from build123d import *

# Parameters (mm, degrees)
BOSS_EXTRUDE1_DEPTH = 12
BOSS_EXTRUDE2_DEPTH = 3
FILLET1_R           = 1
SKETCH3_R           = 1.75
CUT_EXTRUDE2_DEPTH  = 3


with BuildPart() as part:
    # Sketch1 → Boss-Extrude1 (new body)
    with BuildSketch(Plane.XY):
        Polygon((-30.5, 3), (-18.5, 3), (-18.5, 15), (18.5, 15), (18.5, 3), (30.5, 3), (30.5, 0), (15.5, 0), (15.5, 12), (-15.5, 12), (-15.5, 0), (-30.5, 0), align=None)
    extrude(amount=-BOSS_EXTRUDE1_DEPTH)

    # Sketch2 → Boss-Extrude2 (add)
    with BuildSketch(Plane.XY):
        Polygon((-18.5, 15), (-10.5, 15), (-10.5, 0), (-30.5, 0), (-30.5, 3), (-18.5, 3), align=None)
        Polygon((30.5, 0), (10.5, 0), (10.5, 15), (18.5, 15), (18.5, 3), (30.5, 3), align=None)
    extrude(amount=BOSS_EXTRUDE2_DEPTH)

    # Fillet1
    fillet1_edges = [part.edges().sort_by_distance(p)[0] for p in [
        (-15.5, 6, -12),
        (-30.5, 3, -4.5),
        (-18.5, 3, -4.5),
        (-18.5, 15, -4.5),
        (15.5, 6, -12),
        (18.5, 15, -4.5),
        (18.5, 3, -4.5),
        (30.5, 3, -4.5),
        (30.5, 1.5, -12),
        (24.5, 3, -12),
        (18.5, 9, -12),
        (-10.5, 15, 1.5),
        (-18.5, 9, 3),
        (-24.5, 3, 3),
        (-30.5, 1.5, 3),
        (-10.5, 7.5, 3),
        (-14.5, 15, 3),
        (0, 15, -12),
        (-18.5, 9, -12),
        (-24.5, 3, -12),
        (-30.5, 1.5, -12),
        (0, 15, 0),
        (10.5, 15, 1.5),
        (30.5, 1.5, 3),
        (24.5, 3, 3),
        (18.5, 9, 3),
        (14.5, 15, 3),
        (10.5, 7.5, 3),
    ]]
    fillet(fillet1_edges, radius=FILLET1_R)

    # Sketch3 → Cut-Extrude2 (cut)
    with BuildSketch(Plane(origin=(0, 3, 0), x_dir=(1, 0, 0), z_dir=(0, 1, 0))):
        with Locations((-24.5, 4.5)):
            Circle(SKETCH3_R)
        with Locations((24.5, 4.5)):
            Circle(SKETCH3_R)
    extrude(amount=-CUT_EXTRUDE2_DEPTH, mode=Mode.SUBTRACT)


solid = part.part
Design review of the part built by this model. Coordinates are the model's own, in mm. A direction names the side the tool comes from. Coordinates: 2 decimals unless noted, no trailing zeros. Order: outer loops, then holes, each group sorted by start corner. A loop starts at its lowest first (then second) coordinate and runs counter-clockwise, first axis right, second up.
Item 1: Take a section at D-D, the plane z = -7. Write out the cut boundary in (x, y), then the cut area to 3 significant figures.
Item 2: For faces 1 (the cylindrical face through (-10.801, 14.715, 0.854)), 2 (the cylindrical face through (15.785, 6.084, -11.699)), 3 (the cylindrical face through (18.215, 8.93, 2.699)), 4 (the flat face through (23, 3, -3)), list the 3-axis set-ups (+Z, -Z, +X, -X, +Y, -Y) from which the entire face can be reached by the end or side of a thin tool; tool diameter is ignored.
Item 3: For pin 1 Ø1 at (x, y) = (-1, 12.5) entering from +Z; pin 2 Ø4 at (y, z) = (8, -5) entering from +X; pin 3 Ø5 at (y, z) = (8, 1.5) entering from -X; pin 4 Ø3 at (x, z) = (24.5, -4.5) entering from +Y, all flat-tipped, find the tip position at first contact; note any pin that passes through.
Item 4: Take a section at C-C, the plane x = 24.5. Write out the cut boundary in (y, z).
Item 5: Take a section at A-A, the plane z = -4.5. Write out the cut boundary in (x, y), then the cut area to 3 significant figures.
Item 6: Take a section at B-B, the plane y = 5.75. Write out the cut boundary in (x, z), then the cut area to 3 significant figures.
Item 7: The part is to be moulded in two halves that separate along X. For faces 5 (the cylindrical face through (24.57, 2.715, -11.699)), 6 (the cylindrical face through (-18.215, 9.07, 2.699)), 7 (the flat face through (0, 12, -6)), say which applies: pulls with the +X half, pulls with the -X half, needs draft (parallel to the pull), parting line crosses it, or undercut.
Item 8: For line 1 (X direction, y = 0.8, z = -4.5); line 2 (Z direction, x = 24.5, y = 0.9); line 3 (X direction, y = 9.5, z = 1.5), list the stretches that pass through material, from the lowest coordinate up.
The answers:
1. outline: (-30.5, 0) - (-15.5, 0) - (-15.5, 12) - (15.5, 12) - (15.5, 0) - (30.5, 0) - (30.5, 2) arc R1 ccw to (29.5, 3) - (19.5, 3) arc R1 cw to (18.5, 4) - (18.5, 14) arc R1 ccw to (17.5, 15) - (-17.5, 15) arc R1 ccw to (-18.5, 14) - (-18.5, 4) arc R1 cw to (-19.5, 3) - (-29.5, 3) arc R1 ccw to (-30.5, 2) - close
1. area: 255 mm2
2. face 1: +Z, +Y
2. face 2: -Z, -Y
2. face 3: +Z, +X, +Y
2. face 4: +Z, -Z, +X, +Y
3. pin 1: stops at z = 0
3. pin 2: stops at x = 18.5
3. pin 3: stops at x = -18.5
3. pin 4: passes through
4. outline: (0, -12) - (2, -12) arc R1 ccw to (3, -11) - (3, -6.25) - (0, -6.25) - close; (0, -2.75) - (3, -2.75) - (3, 2) arc R1 ccw to (2, 3) - (0, 3) - close
5. outline: (-30.5, 0) - (-26.25, 0) - (-26.25, 3) - (-29.5, 3) arc R1 ccw to (-30.5, 2) - close; (-22.75, 0) - (-15.5, 0) - (-15.5, 12) - (15.5, 12) - (15.5, 0) - (22.75, 0) - (22.75, 3) - (19.5, 3) arc R1 cw to (18.5, 4) - (18.5, 14) arc R1 ccw to (17.5, 15) - (-17.5, 15) arc R1 ccw to (-18.5, 14) - (-18.5, 4) arc R1 cw to (-19.5, 3) - (-22.75, 3) - close; (26.25, 0) - (30.5, 0) - (30.5, 2) arc R1 ccw to (29.5, 3) - (26.25, 3) - close
5. area: 234 mm2
6. outline: (-18.5, -11) arc R1 ccw to (-17.5, -12) - (-16.5, -12) arc R1 ccw to (-15.5, -11) - (-15.5, 0) - (-10.5, 0) - (-10.5, 2) arc R1 ccw to (-11.5, 3) - (-17.5, 3) arc R1 ccw to (-18.5, 2) - close; (10.5, 0) - (15.5, 0) - (15.5, -11) arc R1 ccw to (16.5, -12) - (17.5, -12) arc R1 ccw to (18.5, -11) - (18.5, 2) arc R1 ccw to (17.5, 3) - (11.5, 3) arc R1 ccw to (10.5, 2) - close
6. area: 118 mm2
7. face 5: needs draft
7. face 6: pulls with the -X half
7. face 7: undercut
8. line 1: x = -30.5 to -26.25, -22.75 to -15.5, 15.5 to 22.75, 26.25 to 30.5
8. line 2: z = -12 to -6.25, -2.75 to 3
8. line 3: x = -18.5 to -10.5, 10.5 to 18.5
